from build123d import *

# Parameters (mm, degrees)
SKETCH1_R           = 2.1
BOSS_EXTRUDE1_DEPTH = 70
FILLET1_R           = 0.5
CUT_EXTRUDE1_DEPTH  = 72.414284285


with BuildPart() as part:
    # Sketch1 → Boss-Extrude1 (new body)
    with BuildSketch(Plane.XY):
        Polygon((-10, 10), (-4.775, 10), (-3.1, 8.325), (-5.5, 8.325), (-5.5, 6.525), (-3, 4.025), (3, 4.025), (5.5, 6.525), (5.5, 8.325), (3.1, 8.325), (4.775, 10), (10, 10), (10, 4.775), (8.325, 3.1), (8.325, 5.5), (6.525, 5.5), (4.025, 3), (4.025, -3), (6.525, -5.5), (8.325, -5.5), (8.325, -3.1), (10, -4.775), (10, -10), (4.775, -10), (3.1, -8.325), (5.5, -8.325), (5.5, -6.525), (3, -4.025), (-3, -4.025), (-5.5, -6.525), (-5.5, -8.325), (-3.1, -8.325), (-4.775, -10), (-10, -10), (-10, -4.775), (-8.325, -3.1), (-8.325, -5.5), (-6.525, -5.5), (-4.025, -3), (-4.025, 3), (-6.525, 5.5), (-8.325, 5.5), (-8.325, 3.1), (-10, 4.775), align=None)
        Circle(SKETCH1_R, mode=Mode.SUBTRACT)
    extrude(amount=BOSS_EXTRUDE1_DEPTH)

    # Fillet1
    fillet1_edges = [part.edges().sort_by_distance(p)[0] for p in [
        (10, -10, 35),
        (-10, -10, 35),
        (-10, 10, 35),
        (10, 10, 35),
    ]]
    fillet(fillet1_edges, radius=FILLET1_R)

    # Sketch2 → Cut-Extrude1 (cut, through all)
    with BuildSketch(Plane.XY.offset(70)):
        with BuildLine():
            ThreePointArc((-4.025, 0.4), (-4.425, 0), (-4.025, -0.4))
            Line((-4.025, -0.4), (-4.025, 0.4))
        make_face()
        with BuildLine():
            Line((-4.025, 0.4), (-4.025, -0.4))
            ThreePointArc((-4.025, -0.4), (-3.742157288, -0.282842712), (-3.625, 0))
            ThreePointArc((-3.625, 0), (-3.742157288, 0.282842712), (-4.025, 0.4))
        make_face()
        with BuildLine():
            ThreePointArc((0.4, 4.025), (0, 4.425), (-0.4, 4.025))
            Line((-0.4, 4.025), (0.4, 4.025))
        make_face()
        with BuildLine():
            Line((0.4, 4.025), (-0.4, 4.025))
            ThreePointArc((-0.4, 4.025), (0, 3.625), (0.4, 4.025))
        make_face()
        with BuildLine():
            ThreePointArc((4.025, 0.4), (3.625, 0), (4.025, -0.4))
            Line((4.025, -0.4), (4.025, 0.4))
        make_face()
        with BuildLine():
            Line((4.025, 0.4), (4.025, -0.4))
            ThreePointArc((4.025, -0.4), (4.307842712, -0.282842712), (4.425, 0))
            ThreePointArc((4.425, 0), (4.307842712, 0.282842712), (4.025, 0.4))
        make_face()
        with BuildLine():
            ThreePointArc((0.4, -4.025), (0, -3.625), (-0.4, -4.025))
            Line((-0.4, -4.025), (0.4, -4.025))
        make_face()
        with BuildLine():
            Line((0.4, -4.025), (-0.4, -4.025))
            ThreePointArc((-0.4, -4.025), (0, -4.425), (0.4, -4.025))
        make_face()
    extrude(amount=-CUT_EXTRUDE1_DEPTH, mode=Mode.SUBTRACT)


solid = part.part
Model file for the job. Use its own axes, mm. A direction names the side the tool comes from. Round coordinates to 2 decimals unless told otherwise and drop trailing zeros. Write each question's results on one line, items separated by ' | '. Start each with the question number.
(1) Two-plate mould, pull along Y, no slides. Class faces 1 (the face through (7, -10, 35)), 2 (the face through (10, 7, 35)), 3 (the face through (8.325, 4, 35)): pulls with the +Y half, pulls with the -Y half, needs draft (parallel to the pull), parting line crosses it, or undercut.
(2) Drop flat-ended pins along their axis: pin 1 (0.8 mm diameter, centred on y = 2, z = 35, fed in from -X) (3 decimals); pin 2 (0.7 mm diameter, centred on x = -4, z = 46, fed in from -Y) (3 decimals); pin 3 (2 mm diameter, centred on x = -4.5, y = -1, fed in from -Z); pin 4 (3 mm diameter, centred on x = -2, z = 25, fed in from -Y) (3 decimals). Give the stop position or say it passes through.
(3) Probe probe 1 along Y at (x, z) = (0, 39) (3 decimals); probe 2 along Y at (x, z) = (9.25, 33) (3 decimals); probe 3 along Y at (x, z) = (-4.25, 39) (3 decimals). List the from-to ranges inside material, lowest first. Write a range as from..to.
(4) Which spindle directions (+Z, -Z, +X, -X, +Y, -Y) get a long thin tool onto all of the face, cutting with end or side? Do faces 4 (the face through (-3.949, 9.174, 34.51)), 5 (the face through (-9.174, -3.949, 34.51)), 6 (the face through (-8.325, -4, 35)), 7 (the face through (9.151, -3.926, 34.51)), 8 (the face through (3.949, -9.174, 34.51)). Say none if no direction does.
Established:
1) face 1: pulls with the -Y half | face 2: needs draft | face 3: undercut
2) pin 1: stops at x = -4.025 | pin 2: stops at y = -9.575 | pin 3: stops at z = 0 | pin 4: stops at y = -8.725
3) probe 1: y = -3.625..-2.1, 2.1..3.625 | probe 2: y = -10..-4.025, 4.025..10 | probe 3: y = -9.475..-8.325, -5.275..-3.225, 3.225..5.275, 8.325..9.475
4) face 4: +Z, -Z, +Y | face 5: +Z, -Z, -X | face 6: +Z, -Z | face 7: +Z, -Z, +X | face 8: +Z, -Z, -Y
